Read the model definition and answer for the solid it produces. Units are mm, in the model's axes. A direction names the side the tool comes from. Round coordinates to 2 decimals unless told otherwise and drop trailing zeros. Write each loop counter-clockwise with the first axis right and the second up, starting at its lowest first coordinate (ties: lowest second). Pieces come first, ordered by that corner, then holes. Notation, with made-up numbers: (-21.5, 26.5) - (-17.5, 26.5) arc R27 ccw to (-17.5, 63.5) - close; hole circle Ø6 at (77.25, 18.5). An arc over 180 degrees is marked (long way). One line per item, written item: value. Start each with the question number.
(1) The mould has two halves that part along Y. Classify faces 3 (the face through (0.49, -11.99, 0.53)), 4 (the face through (1, -2, 9)), 5 (the face through (4.56, -1.73, -7.81)): +Y half, -Y half, draft (parallel to the pull), parting line (faces both ways), or undercut.
(2) A cutting plane is placed at A-A, the plane z = 0. Determine the outline of the cut face in (x, y).
(3) A cutting plane is placed at C-C, the plane x = 3.25. Determine the outline of the cut face in (y, z), plus the area to 3 significant figures.
(4) For faces 1 (the face through (4.55, -1.172, 8.923)), 2 (the face through (0, 2, -8)), determine the directions among +Z, -Z, +X, -X, +Y, -Y from which every point of the face is accessible in a straight line to the end or side of a thin tool.
(5) A cutting plane is placed at D-D, the plane z = -10.5. Determine the outline of the cut face in (x, y).
(6) Flat-ended cylindrical pins translate along their axes: pin 1 Ø2 at (x, y) = (7.5, 0) entering from +Z; pin 2 Ø1.5 at (x, y) = (6.5, 8.5) entering from -Z; pin 3 Ø5 at (x, z) = (2.5, 7.5) entering from -Y; pin 4 Ø13 at (y, z) = (0, 0) entering from +X. Find the tip coordinate at first contact, or state that the pin passes through.
(7) Find the intervals of material crossed by L1, parallel to Z at x = 6.75, y = 0; L2, parallel to X at y = -4.75, z = 8.5; L3, parallel to Z at x = 6.25, y = 4.75, in increasing order.
from build123d import *

# Parameters (mm, degrees)
SFAZOWANIE1_SIZE  = 0.8
SFAZOWANIE1_SIZE2 = 0.461880215


with BuildPart() as part:
    # Szkic1 → Obrót1 (revolve)
    with BuildSketch(Plane.XY):
        Polygon((0, 8), (9, 8), (9, 9), (1, 9), (1, 12), (0, 12), align=None)
    revolve(axis=Axis((0, 0, 0), (1, 0, 0)))

    # Sfazowanie1
    sfazowanie1_edges = [part.edges().sort_by_distance(p)[0] for p in [
        (9, -9, 0),
    ]]
    sfazowanie1_side = [part.faces().sort_by_distance(p)[0] for p in [
        (5, -9, 0),
    ]]
    chamfer(sfazowanie1_edges, length=SFAZOWANIE1_SIZE, length2=SFAZOWANIE1_SIZE2, reference=sfazowanie1_side[0])


solid = part.part
Here are the results:
1. face 3: parting line
1. face 4: draft
1. face 5: undercut
2. outline: (0, -12) - (1, -12) - (1, -9) - (8.2, -9) - (9, -8.54) - (9, -8) - (0, -8) - close; (0, 8) - (9, 8) - (9, 8.54) - (8.2, 9) - (1, 9) - (1, 12) - (0, 12) - close
3. outline: circle Ø18 at (0, 0); hole circle Ø16 at (0, 0)
3. area: 53.4 mm²
4. face 1: +X
4. face 2: +Z, -Z, -X, +Y, -Y
5. outline: (0, -5.81) - (1, -5.81) - (1, 5.81) - (0, 5.81) - close
6. pin 1: z = 9
6. pin 2: z = -4.58
6. pin 3: y = -10.67
6. pin 4: through
7. L1: -9 to -8, 8 to 9
7. L2: 0 to 1
7. L3: -7.64 to -6.44, 6.44 to 7.64
